Could you check a few things on this model? Use its own coordinates, in mm. Face numbers are marked on the shaded views. A direction names the side the tool comes from. Round coordinates to 2 decimals unless told otherwise and drop trailing zeros. Write each loop counter-clockwise with the first axis right and the second up, starting at its lowest first coordinate (ties: lowest second). Pieces come first, ordered by that corner, then holes. Notation, with made-up numbers: (80.25, 88) - (135.25, 88) arc R19 cw to (135.25, 113) - close; hole circle Ø10 at (69.5, 67). An arc over 180 degrees is marked (long way). Write each question's results on one line, items separated by ' | '. Start each with the question number.
(1) Please list where these lines run through material, in increasing order: line 1 (X direction, y = -4, z = -13); line 2 (Y direction, x = -21, z = -15); line 3 (Z direction, x = -27, y = 10). Write a range as [from, to].
(2) On a 3-axis mill with a long thin cutter (end or side, diameter ignored), from which of +Z, -Z, +X, -X, +Y, -Y can I reach the whole of each face in a straight line? I mean the marked faces 1, 2 and 3. Say none if no direction works.
(3) Imagine slicing it at B-B on z = -12. Write out the boundary of the cut face in (x, y), then the cut area to 3 significant figures.
(4) Thinking about a two-plate mould opening in X: for the marked faces 4, 5, 6 and 7, which applies, +X half, -X half, draft (parallel to the pull), parting line (faces both ways), or undercut?
(5) Imagine slicing it at A-A on y = 0. Write out the boundary of the cut face in (x, z).
(6) For P1, Ø3, axis at x = -36.25, y = 0, coming from the -Z side; P2, Ø4, axis at x = 29.5, z = -11, coming from the +Y side; P3, Ø2, axis at y = 6, z = -28, coming from the +X side; P4, Ø3, axis at x = -10, y = 8.5, coming from the +Z side, each with a flat end and sliding along its axis, tell me the tip position at first contact or that it passes through.
(7) Imagine slicing it at D-D on y = 9.5. Write out the boundary of the cut face in (x, z).
(8) Imagine slicing it at C-C on x = 12.5. Write out the boundary of the cut face in (y, z), then the cut area to 3 significant figures.
```python
from build123d import *

# Parameters (mm, degrees)
SCHIZZO1_R                   = 1.7
ESTRUSIONE_ESTRUSIONE1_DEPTH = 4.1
SCHIZZO2_W                   = 65.5
SCHIZZO2_H                   = 32
SCHIZZO2_W_2                 = 63.5
SCHIZZO2_H_2                 = 30
ESTRUSIONE_SOTTILE1_DEPTH    = 35
SMUSSO1_SIZE                 = 1.5


with BuildPart() as part:
    # Schizzo1 → Estrusione-Estrusione1 (new body)
    with BuildSketch(Plane.XY):
        with BuildLine():
            Line((32.14828078, 18), (-32.14828078, 18))
            ThreePointArc((-32.14828078, 18), (-35.199603729, 16.960988294), (-36.982782572, 14.275771306))
            Line((-36.982782572, 14.275771306), (-40.076676255, 2.551542612))
            ThreePointArc((-40.076676255, 2.551542612), (-40.407672672, 0), (-40.076676255, -2.551542612))
            Line((-40.076676255, -2.551542612), (-36.982782572, -14.275771306))
            ThreePointArc((-36.982782572, -14.275771306), (-35.199603729, -16.960988294), (-32.14828078, -18))
            Line((-32.14828078, -18), (32.14828078, -18))
            ThreePointArc((32.14828078, -18), (35.199603729, -16.960988294), (36.982782572, -14.275771306))
            Line((36.982782572, -14.275771306), (40.076676255, -2.551542612))
            ThreePointArc((40.076676255, -2.551542612), (40.407672672, 0), (40.076676255, 2.551542612))
            Line((40.076676255, 2.551542612), (36.982782572, 14.275771306))
            ThreePointArc((36.982782572, 14.275771306), (35.199603729, 16.960988294), (32.14828078, 18))
        make_face()
        with Locations((-36.25, 0)):
            Circle(SCHIZZO1_R, mode=Mode.SUBTRACT)
        with Locations((36.25, 0)):
            Circle(SCHIZZO1_R, mode=Mode.SUBTRACT)
    extrude(amount=-ESTRUSIONE_ESTRUSIONE1_DEPTH)

    # Schizzo2 → Estrusione-Sottile1 (add)
    with BuildSketch(Plane(origin=(0, 0, -4.1), x_dir=(-1, 0, 0), z_dir=(0, 0, -1))):
        Rectangle(SCHIZZO2_W, SCHIZZO2_H)
        Rectangle(SCHIZZO2_W_2, SCHIZZO2_H_2, mode=Mode.SUBTRACT)
    extrude(amount=ESTRUSIONE_SOTTILE1_DEPTH)

    # Smusso1
    smusso1_edges = [part.edges().sort_by_distance(p)[0] for p in [
        (-37.95, 0, 0),
        (34.55, 0, 0),
    ]]
    chamfer(smusso1_edges, length=SMUSSO1_SIZE)


solid = part.part
```
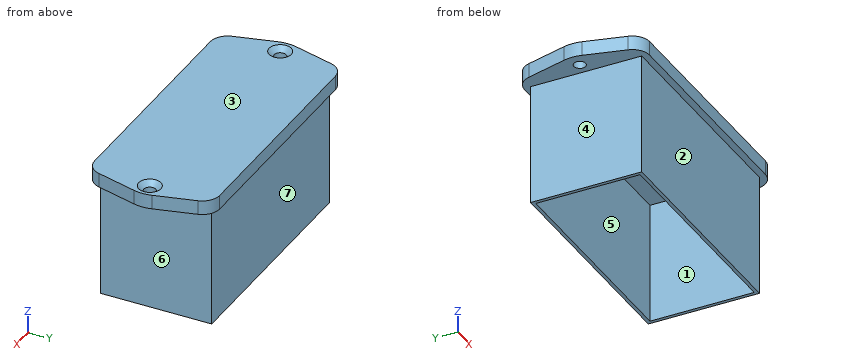
Response:
1) line 1: [-32.75, -31.75], [31.75, 32.75] | line 2: [-16, -15], [15, 16] | line 3: [-4.1, 0]
2) face 1: -Z | face 2: -Z, +X, -X, -Y | face 3: +Z, +X, -X, +Y, -Y
3) outline: (-32.75, -16) - (32.75, -16) - (32.75, 16) - (-32.75, 16) - close; hole (-31.75, -15) - (31.75, -15) - (31.75, 15) - (-31.75, 15) - close | area: 191 mm²
4) face 4: -X half | face 5: undercut | face 6: +X half | face 7: draft
5) outline: (-40.41, -4.1) - (-37.95, -4.1) - (-37.95, -1.5) - (-39.45, 0) - (-40.41, 0) - close; (-34.55, -4.1) - (-32.75, -4.1) - (-32.75, -39.1) - (-31.75, -39.1) - (-31.75, -4.1) - (31.75, -4.1) - (31.75, -39.1) - (32.75, -39.1) - (32.75, -4.1) - (34.55, -4.1) - (34.55, -1.5) - (33.05, 0) - (-33.05, 0) - (-34.55, -1.5) - close; (37.95, -4.1) - (40.41, -4.1) - (40.41, 0) - (39.45, 0) - (37.95, -1.5) - close
6) P1: through | P2: y = 16 | P3: x = 32.75 | P4: z = 0
7) outline: (-38.24, -4.1) - (-32.75, -4.1) - (-32.75, -39.1) - (-31.75, -39.1) - (-31.75, -4.1) - (31.75, -4.1) - (31.75, -39.1) - (32.75, -39.1) - (32.75, -4.1) - (38.24, -4.1) - (38.24, 0) - (-38.24, 0) - close
8) outline: (-18, -4.1) - (-16, -4.1) - (-16, -39.1) - (-15, -39.1) - (-15, -4.1) - (15, -4.1) - (15, -39.1) - (16, -39.1) - (16, -4.1) - (18, -4.1) - (18, 0) - (-18, 0) - close | area: 218 mm²
